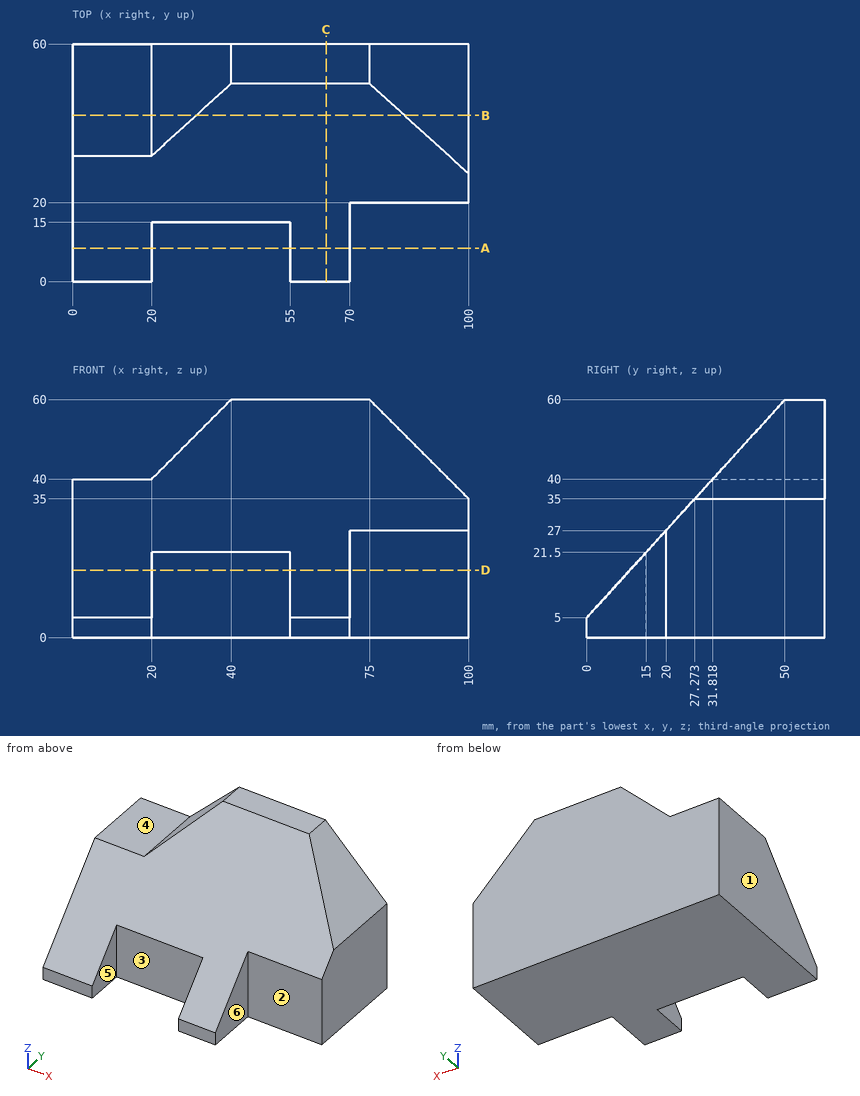
Could you check a few things on this drawing? It's one solid part, dimensions in mm from its lowest x, y, z. A direction names the side the tool comes from. Give positions to 0.01 mm unless a question says otherwise; leave off trailing zeros. Loops run counter-clockwise (first coordinate to the right, second up) from the corner with the lowest first, then second, coordinate; pieces in that order, holes last. Notation, with made-up numbers: M -39,-26.5 L 17,-26.5 A23 cw 17,12.5 Z; hole C -15,-20 d6. An arc over 180 degrees is marked long. Answer as a JSON object with one key per item and string values.
Q1. For P1, Ø12, axis at x = 85, y = 49.5, coming from the +Z side; P2, Ø22, axis at y = 7.5, z = 12, coming from the +X side; P3, Ø8, axis at y = 46, z = 44.5, coming from the -X side, each with a flat end and sliding along its axis, tell me the tip position at first contact or that it passes through.
Values found:
{"P1": "stops at z = 56", "P2": "stops at x = 70", "P3": "stops at x = 20.5"}
Q2. Suppose I cut it at C-C, the plane x = 64. List the corners of the cut face in (y, z) for me.
Values found:
{"outline": "M 0,0 L 60,0 L 60,60 L 50,60 L 0,5 Z"}
Q3. If we mould it in two halves opening along X, with no side actions, what happens to the marked faces 4, 5 and 6? For each: pulls with the +X half, pulls with the -X half, needs draft (parallel to the pull), parting line crosses it, or undercut.
Values found:
{"face 4": "needs draft", "face 5": "undercut", "face 6": "pulls with the +X half"}
Q4. For the marked faces 1, 2 and 3, which set-ups out of +Z, -Z, +X, -X, +Y, -Y let a thin tool reach every point of the face, with its end or its side?
Values found:
{"face 1": "+Z, -Z, -X, +Y, -Y", "face 2": "+Z, -Z, +X, -Y", "face 3": "+Z, -Z, -Y"}
Q5. Suppose I cut it at B-B, the plane y = 42. List the corners of the cut face in (x, z) for me, plus the area to 3 significant figures.
Values found:
{"outline": "M 0,0 L 100,0 L 100,35 L 83.8,51.2 L 31.2,51.2 L 20,40 L 0,40 Z", "area": "4,700 mm²"}
Q6. Suppose I cut it at A-A, the plane y = 8.5. List the corners of the cut face in (x, z) for me, plus the area to 3 significant figures.
Values found:
{"outline": "M 0,0 L 20,0 L 20,14.35 L 0,14.35 Z; M 55,0 L 70,0 L 70,14.35 L 55,14.35 Z", "area": "502 mm²"}
Q7. If I drill on probe 1 along X at (y, z) = (12, 13); probe 2 along Y at (x, z) = (57, 49); probe 3 along Y at (x, z) = (92, 23), over which ranges is the centre line in solid material (lowest first)? Write a range as [from, to].
Values found:
{"probe 1": "x = [0, 20], [55, 70]", "probe 2": "y = [40, 60]", "probe 3": "y = [20, 60]"}
Q8. Suppose I cut it at D-D, the plane z = 17. List the corners of the cut face in (x, y) for me.
Values found:
{"outline": "M 0,10.91 L 20,10.91 L 20,15 L 55,15 L 55,10.91 L 70,10.91 L 70,20 L 100,20 L 100,60 L 0,60 Z"}
